from build123d import *

# Parameters (mm, degrees)
F1_DEPTH = 10


with BuildPart() as f1:
    # F0 (on Top) → F1 (new body)
    with BuildSketch(Plane.XY):
        with BuildLine():
            Line((-17.0999729578, 13.9659811929), (-29.5999729578, 13.9659811929))
            Line((-29.5999729578, 13.9659811929), (-29.5999729578, 6.4659811929))
            Line((-29.5999729578, 6.4659811929), (-26.3499729578, 6.4659811929))
            ThreePointArc((-26.3499729578, 6.4659811929), (-25.0999729578, 7.7159811929), (-23.8499729578, 6.4659811929))
            Line((-23.8499729578, 6.4659811929), (-17.0999729578, 6.4659811929))
            Line((-17.0999729578, 6.4659811929), (-17.0999729578, 13.9659811929))
        make_face()
        with BuildLine():
            Line((-4.5999729578, 13.9659811929), (-17.0999729578, 13.9659811929))
            Line((-17.0999729578, 13.9659811929), (-17.0999729578, 6.4659811929))
            Line((-17.0999729578, 6.4659811929), (-10.3499729578, 6.4659811929))
            ThreePointArc((-10.3499729578, 6.4659811929), (-9.0999729578, 7.7159811929), (-7.8499729578, 6.4659811929))
            Line((-7.8499729578, 6.4659811929), (-4.5999729578, 6.4659811929))
            Line((-4.5999729578, 6.4659811929), (-4.5999729578, 13.9659811929))
        make_face()
    extrude(amount=F1_DEPTH)


solid = f1.part
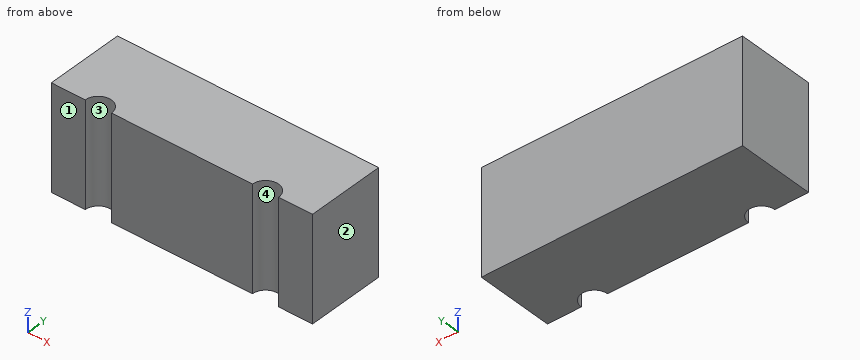
The listing builds one solid part. Answer for the finished solid, in the listing's coordinates (mm). Face numbers are marked on the shaded views. Coordinates: 2 decimals unless noted, no trailing zeros. Order: outer loops, then holes, each group sorted by start corner. A loop starts at its lowest first (then second) coordinate and runs counter-clockwise, first axis right, second up. Notation, with made-up numbers: M -27.75,30.25 L -6.75,30.25 A18 cw -6.75,49.25 Z; hole C 65.5,4.25 d6. An arc over 180 degrees is marked long. Use CSV: the item, a comma, the result in double quotes.
Q1. Section B-B (z = 4.5) is taken. Determine the outline of the cut face in (x, y).
Here are the results:
outline,"M -29.6,6.47 L -26.35,6.47 A1.25 cw -23.85,6.47 L -10.35,6.47 A1.25 cw -7.85,6.47 L -4.6,6.47 L -4.6,13.97 L -29.6,13.97 Z"
Q2. A straight line is drawn through the part: L1, parallel to Y at x = -8.5, z = 5.25. Find the intervals that lie inside material, in ascending order.
Here are the results:
L1,"7.56 to 13.97"
Q3. Section A-A (y = 7) is taken. Determine the outline of the cut face in (x, z).
Here are the results:
outline,"M -29.6,0 L -26.23,0 L -26.23,10 L -29.6,10 Z; M -23.97,0 L -10.23,0 L -10.23,10 L -23.97,10 Z; M -7.97,0 L -4.6,0 L -4.6,10 L -7.97,10 Z"
Q4. Determine the mould class of the marked faces 1, 2, 3 and 4 for opening direction X: pulls with the +X half, pulls with the -X half, needs draft (parallel to the pull), parting line crosses it, or undercut.
Here are the results:
face 1,"needs draft"
face 2,"pulls with the +X half"
face 3,"undercut"
face 4,"undercut"
